```python
from build123d import *

# Parameters (mm, degrees)
F1_DEPTH = 30
F2_R     = 1


with BuildPart() as f1:
    # F0 (on Top) → F1 (new body)
    with BuildSketch(Plane.XY):
        Polygon((10, 0), (5, 8.660254), (-5, 8.660254), (-10, 0), (-5, -8.660254), (5, -8.660254), align=None)
        Polygon((3.267949, -5.660254), (-3.267949, -5.660254), (-6.535898, 0), (-3.267949, 5.660254), (3.267949, 5.660254), (6.535898, 0), align=None, mode=Mode.SUBTRACT)
    extrude(amount=F1_DEPTH)

    # F2
    f2_edges = [f1.edges().sort_by_distance(p)[0] for p in [
        (-5, -8.660254, 15),
        (0, -8.660254, 30),
        (5, -8.660254, 15),
        (7.5, -4.330127, 30),
        (10, 0, 15),
        (7.5, 4.330127, 30),
        (5, 8.660254, 15),
        (0, 8.660254, 30),
        (-5, 8.660254, 15),
        (-7.5, 4.330127, 30),
        (-10, 0, 15),
        (-7.5, -4.330127, 30),
    ]]
    fillet(f2_edges, radius=F2_R)


solid = f1.part
```
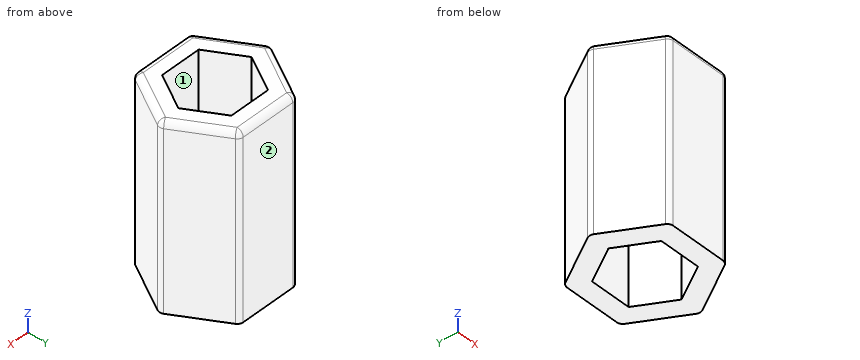
Work out the finished part from the listing and answer in its coordinate system (mm). Face numbers are marked on the shaded views. A direction names the side the tool comes from. Round coordinates to 2 decimals unless told otherwise and drop trailing zeros. Loops run counter-clockwise (first coordinate to the right, second up) from the corner with the lowest first, then second, coordinate; pieces in that order, holes last.
(1) For the marked faces 1 and 2, determine the directions among +Z, -Z, +X, -X, +Y, -Y from which every point of the face is accessible in a straight line to the end or side of a thin tool.
Computed values:
face 1: +Z, -Z
face 2: +Z, -Z, +X, -X, +Y
(2) Each of these flat-tipped pins is pushed along its axis until it touches: P1, Ø1, axis at y = -1, z = 7.5, coming from the -X side; P2, Ø1, axis at y = -3.5, z = 22, coming from the +X side. Where does it stop, or does it pass through?
Computed values:
P1: stops at x = -9.71
P2: stops at x = 8.27
(3) Find the intervals of material crossed by L1, parallel to Y at x = -2, z = 20.5; L2, parallel to Z at x = -4.5, y = 7.75; L3, parallel to Y at x = -4.5, z = 22, in increasing order.
Computed values:
L1: y = -8.66 to -5.66, 5.66 to 8.66
L2: z = 0 to 29.99
L3: y = -8.66 to -3.53, 3.53 to 8.66
(4) The part is cut by section A-A, the plane z = 6. Give the vertices of the cut face in (x, y).
Computed values:
outline: (-9.71, -0.5) - (-5.29, -8.16) arc R1 ccw to (-4.42, -8.66) - (4.42, -8.66) arc R1 ccw to (5.29, -8.16) - (9.71, -0.5) arc R1 ccw to (9.71, 0.5) - (5.29, 8.16) arc R1 ccw to (4.42, 8.66) - (-4.42, 8.66) arc R1 ccw to (-5.29, 8.16) - (-9.71, 0.5) arc R1 ccw to start; hole (-6.54, 0) - (-3.27, -5.66) - (3.27, -5.66) - (6.54, 0) - (3.27, 5.66) - (-3.27, 5.66) - close
